from build123d import *

# Parameters (mm, degrees)
SKETCH1_R           = 1.75
BOSS_EXTRUDE1_DEPTH = 11
FILLET1_R           = 1.75
SKETCH3_W           = 5
SKETCH3_H           = 5
BOSS_EXTRUDE2_DEPTH = 3


with BuildPart() as part:
    # Sketch1 → Boss-Extrude1 (new body)
    with BuildSketch(Plane(origin=(0, 0, 0), x_dir=(1, 0, 0), z_dir=(0, 1, 0))):
        with Locations(Location((0, 0, 0), (0, 0, 270))):
            Circle(SKETCH1_R)
    extrude(amount=BOSS_EXTRUDE1_DEPTH)

    # Fillet1
    fillet1_edges = [part.edges().sort_by_distance(p)[0] for p in [
        (0, 11, -1.75),
    ]]
    fillet(fillet1_edges, radius=FILLET1_R)

    # Sketch3 → Boss-Extrude2 (add)
    with BuildSketch(Plane.XZ):
        Rectangle(SKETCH3_W, SKETCH3_H)
    extrude(amount=-BOSS_EXTRUDE2_DEPTH)


solid = part.part
Read the model definition and answer for the solid it produces. Units are mm, in the model's axes. A direction names the side the tool comes from. Round coordinates to 2 decimals unless told otherwise and drop trailing zeros. Loops run counter-clockwise (first coordinate to the right, second up) from the corner with the lowest first, then second, coordinate; pieces in that order, holes last. Notation, with made-up numbers: (18.5, 29) - (44.5, 29) arc R36 cw to (44.5, 66) - close; hole circle Ø11 at (-27, 76). An arc over 180 degrees is marked (long way). One line per question, with ' | ' between items. Start each with the question number.
Q1. Find the intervals of material crossed by L1, parallel to Y at x = 1.8, z = -1.05; L2, parallel to Z at x = -0.05, y = 7.5; L3, parallel to Y at x = -0.75, z = -0.3, in increasing order.
Q2. Section C-C on y = 5 is taken. Give the vertices of the cut face in (x, z).
Q3. Section A-A on z = 0 is taken. Give the vertices of the cut face in (x, y).
Q4. Flat-ended cylindrical pins translate along their axes: pin 1 (3 mm diameter, centred on y = 9.5, z = 1, fed in from +X); pin 2 (3 mm diameter, centred on x = -1.5, y = 10, fed in from +Z). Find the tip coordinate at first contact, or state that the pin passes through.
Q5. For faces 1 (the flat face through (-1, 3, 2)), 2 (the flat face through (0, 1, 2.5)), determine the directions among +Z, -Z, +X, -X, +Y, -Y from which every point of the face is accessible in a straight line to the end or side of a thin tool.
Q6. Section B-B on x = 0 is taken. Give the vertices of the cut face in (y, z).
Established:
1) L1: 0 to 3 | L2: -1.75 to 1.75 | L3: 0 to 10.8
2) outline: circle Ø3.5 at (0, 0)
3) outline: (-2.5, 0) - (2.5, 0) - (2.5, 3) - (1.75, 3) - (1.75, 9.25) arc R1.75 ccw to (-1.75, 9.25) - (-1.75, 3) - (-2.5, 3) - close
4) pin 1: x = 1.75 | pin 2: z = 1.74
5) face 1: +Y | face 2: +Z, +X, -X, +Y, -Y
6) outline: (0, -2.5) - (3, -2.5) - (3, -1.75) - (9.25, -1.75) arc R1.75 ccw to (9.25, 1.75) - (3, 1.75) - (3, 2.5) - (0, 2.5) - close
